Autodesk Inventor part; units mm, degrees
ref_plane "YZ Plane" through (0, 0, 0) normal (1, 0, 0) x (0, 1, 0)
ref_plane "XZ Plane" through (0, 0, 0) normal (0, 1, 0) x (-1, 0, 0)
ref_plane "XY Plane" through (0, 0, 0) normal (0, 0, 1) x (1, 0, 0)
sketch "Sketch1" plane through (0, 0, 0) normal (0, 0, 1) x (1, 0, 0)
  line L0 (-9.525, -26) -> (9.525, -26)
  line L1 (9.525, -26) -> (9.525, 26)
  line L2 (9.525, 26) -> (-9.525, 26)
  line L3 (-9.525, 26) -> (-9.525, -26)
  line L4 (-9.525, -26) -> (9.525, 26) construction
  line L5 (9.525, -26) -> (-9.525, 26) construction
  point P0 (0, 0)
  dimension "d0" = 19.05
  dimension "d1" = 52
extrude "Extrusion1" add sketch "Sketch1" along normal blind 6.35
sketch "Sketch3" plane through (-9.525, 26, 0) normal (0, 1, 0) x (1, 0, 0)
  line L0 (19.05, 0) -> (0, 0)
  line L1 (0, 0) -> (0, -6.35)
  line L2 (19.05, -6.35) -> (0, -6.35)
  line L3 (19.05, 0) -> (19.05, -6.35)
  line L4 (0, 0) -> (0, -6.35)
  line L5 (0, 0) -> (19.05, -6.35)
  point P0 (9.525, 0)
  point P1 (9.525, -3.175)
hole "Hole1" at (0, 26, 3.175) direction (0, -1, 0) diameter 2.156 depth 8.865 tip angle 118
mirror "Mirror1" about plane through (0, 0, 0) normal (0, 1, 0) of "Hole1"
equation "\"d0\" = sensorHolderDepth"
equation "\"d1\" = detectorWidth"
equation "\"d2\" = acrylicThickness"
equation "\"acrylicThickness\" = 6.35"
equation "\"height\" = 127"
equation "\"width\" = 127"
equation "\"depth\" = 273.05"
equation "\"mirrorAngle\" = 5deg"
equation "\"detectorWidth\" = 52"
equation "\"detectorHeight\" = 52"
equation "\"mirrorThickness\" = 3.175"
equation "\"fresnelThickness\" = 0.1"
equation "\"focalLength\" = 76.2"
equation "\"ior\" = 1.49"
equation "\"centerThickness\" = 1.524"
equation "\"fresnelAngle\" = 90deg"
equation "\"fresnelEffectiveDiameter\" = 152.4"
equation "\"mirrorSuppourtWidth\" = 38.1"
equation "\"backGrooveBit\" = 4.8006"
equation "\"detectorOpeningWidth\" = 76.2"
equation "\"detectorOpeningHeight\" = 76.2"
equation "\"sensorHolderSensorHeight\" = 53.975"
equation "\"sensorHolderSensorWidth\" = 53.975"
equation "\"oRingWidth\" = 1.5875"
equation "\"sensorHolderORingID\" = 203.2"
equation "\"sensorHolderFlushORingID\" = 304.8"
equation "\"frontBackORingID\" = 419.1"
equation "\"mirrorGroove\" = 19.05"
equation "\"backMirrorGroove\" = 6.35"
equation "\"fresnelMirrorChamfer\" = 6.35"
equation "\"mirrorGrooveMill\" = 3.175"
equation "\"sensorHolderDepth\" = 19.05"
equation "\"frameAcrylicThickness\" = 9.525"
equation "\"internalAcrylicThicnkess\" = 6.35"
equation "\"internalAcrylicThickness\" = 6.35"
equation "\"aerogelClearence\" = 3.175"
equation "\"backplanePCBWidth\" = 76.2"
equation "\"backplanePostionOffsett\" = 12.7"
equation "\"backplaneHoleOffsett\" = 6.35"
equation "\"backplanePCBHeight\" = 76.2"
equation "\"moduleSlotClearence\" = 0.79375"
properties part number "detectorSuppourt" material "ABS Plastic"
For this review, take the finished solid that the model builds, in its own axes (mm). A direction names the side the tool comes from. Round coordinates to 2 decimals unless told otherwise and drop trailing zeros. Write each loop counter-clockwise with the first axis right and the second up, starting at its lowest first coordinate (ties: lowest second). Pieces come first, ordered by that corner, then holes. Notation, with made-up numbers: (35, 39.5) -> (79, 39.5) arc R5 cw to (79, 43.5) -> close; hole circle Ø10 at (55.25, 0.5). An arc over 180 degrees is marked (long way). One line per question, with ' | ' between items. Start each with the question number.
(1) For line 1 along Z through (x, y) = (0, 20.5), list the stretches that pass through material, from the lowest coordinate up. Write a range as from..to.
(2) Tool access review of faces 4 (the face through (0.05, -21.51, 2.1)), 5 (the face through (0, 26, 5)): name each direction out of +Z, -Z, +X, -X, +Y, -Y from which nothing blocks a thin tool from reaching the whole face with its end or side.
(3) Add section A-A, the plane y = -20.5. Write out the cut boundary in (x, z) (3 decimals), plus the area to 3 significant figures.
(4) Mouldability with a two-part tool opening along X and no side actions: class faces 1 (the face through (0, 0, 6.35)), 2 (the face through (-0.05, 21.51, 2.1)), 3 (the face through (-9.525, 0, 3)) as released by +X, released by -X, zero draft, split by the parting line, or undercut.
Answer list:
1) line 1: 0..2.1, 4.25..6.35
2) face 4: -Y | face 5: +Z, -Z, +X, -X, +Y
3) outline: (-9.525, 0) -> (9.525, 0) -> (9.525, 6.35) -> (-9.525, 6.35) -> close; hole circle Ø2.156 at (0, 3.175) | area: 117 mm²
4) face 1: zero draft | face 2: undercut | face 3: released by -X
